Part model, mm, in its own coordinate system. Face numbers are marked on the shaded views. A direction names the side the tool comes from. Give positions to 0.01 mm unless a question says otherwise; leave off trailing zeros. Write each loop counter-clockwise with the first axis right and the second up, starting at its lowest first coordinate (ties: lowest second). Pieces come first, ordered by that corner, then holes.
from build123d import *

# Parameters (mm, degrees)
F2_DEPTH    = 10
F3_W        = 20.5154874287
F3_H        = 21.7
F4_DEPTH    = 1
F5_R        = 5
F7_T1_DEPTH = 14.7609215151
F7_T4_ANGLE = 34.9116466648
F7_T6_ANGLE = 279.6444662417
F7_T8_ANGLE = 34.9116520269


# Not quite as in the source:
# - a fillet or chamfer that OpenCascade refuses, or shapes differently, is made with other operations: its cross-section is extruded or revolved along the edge and cut away or added


with BuildPart() as f2:
    # F0 (on Top) → F2 (new body)
    with BuildSketch(Plane.XY):
        with BuildLine():
            ThreePointArc((7.5612498967, -5.5), (-9.35, 0), (7.5612498967, 5.5))
            Line((7.5612498967, 5.5), (8.2899034976, 7))
            ThreePointArc((8.2899034976, 7), (-10.85, 0), (8.2899034976, -7))
            Line((8.2899034976, -7), (7.5612498967, -5.5))
        make_face()
    extrude(amount=F2_DEPTH)

    # F3 (on Top) → F4 (join)
    with BuildSketch(Plane.XY):
        with Locations((-0.5922562857, 0)):
            Rectangle(F3_W, F3_H)
    extrude(amount=F4_DEPTH)

    # F5
    f5_edges = [f2.edges().sort_by_distance(p)[0] for p in [
        (-10.85, -10.85, 0.5),
        (9.665487, -10.85, 0.5),
        (-10.85, 10.85, 0.5),
        (9.665487, 10.85, 0.5),
    ]]
    fillet(f5_edges, radius=F5_R)

    # F7: fillet of radius 2 on 3 edges, made by hand

    # F7_s2 → F7_t1 (cut)
    with BuildSketch(Plane.XY.offset(1)):
        with BuildLine():
            ThreePointArc((8.2899034976, 7), (7.1091806232, 6.7248281543), (5.9864319049, 7.1822790985))
            ThreePointArc((5.9864319049, 7.1822790985), (6.8258652411, 6.3898406639), (7.5612498967, 5.5))
            Line((7.5612498967, 5.5), (8.2899034976, 7))
        make_face()
        with BuildLine():
            ThreePointArc((5.9864319049, -7.1822790985), (7.1091806232, -6.7248281543), (8.2899034976, -7))
            Line((8.2899034976, -7), (7.5612498967, -5.5))
            ThreePointArc((7.5612498967, -5.5), (6.8258652411, -6.3898406639), (5.9864319049, -7.1822790985))
        make_face()
    extrude(amount=F7_T1_DEPTH, mode=Mode.SUBTRACT)

    # F7_s3 → F7_t4 (revolve, cut)
    with BuildSketch(Plane(origin=(0, 0, 0), x_dir=(0, 0, 1), z_dir=(0.091781739, 0.9957791484, 0))):
        with BuildLine():
            ThreePointArc((8, 9.35), (9.4142135624, 9.9357864376), (10, 11.35))
            Line((10, 11.35), (10, 9.35))
            Line((10, 9.35), (8, 9.35))
        make_face()
    revolve(axis=Axis((0, 0, 10), (0, 0, -1)), revolution_arc=F7_T4_ANGLE, mode=Mode.SUBTRACT)

    # F7_s5 → F7_t6 (revolve, cut)
    with BuildSketch(Plane(origin=(0, 0, 0), x_dir=(0, 0, 1), z_dir=(0.6451612191, 0.7640464655, 0))):
        with BuildLine():
            ThreePointArc((8.0635083269, 9.35), (9.2882531983, 9.7688611699), (10, 10.85))
            Line((10, 10.85), (10, 9.35))
            Line((10, 9.35), (8.0635083269, 9.35))
        make_face()
    revolve(axis=Axis((0, 0, 10), (0, 0, -1)), revolution_arc=F7_T6_ANGLE, mode=Mode.SUBTRACT)

    # F7_s7 → F7_t8 (revolve, cut)
    with BuildSketch(Plane(origin=(0, 0, 0), x_dir=(0, 0, 1), z_dir=(-0.6451612906, 0.7640464051, 0))):
        with BuildLine():
            ThreePointArc((8, 9.35), (9.4142135624, 9.9357864376), (10, 11.35))
            Line((10, 11.35), (10, 9.35))
            Line((10, 9.35), (8, 9.35))
        make_face()
    revolve(axis=Axis((0, 0, 10), (0, 0, -1)), revolution_arc=F7_T8_ANGLE, mode=Mode.SUBTRACT)


solid = f2.part
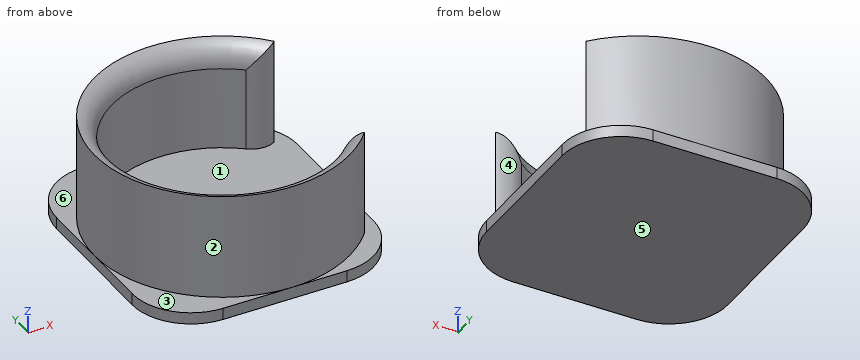
1) Saw through at B-B (z = 9.25). Write the cut outline in (x, y), and give its area (3 significant figures).
Check result:
outline: (7.04, -6.73) arc R9.74 cw (long way) to (7.04, 6.73) arc R2 ccw to (8.29, 7) arc R10.85 ccw (long way) to (8.29, -7) arc R2 ccw to start
area: 55.3 mm2
2) Flat gauge pins, fed straight in: P1, Ø3.5, axis at x = -7, y = 4, coming from the +Z side; P2, Ø1, axis at x = 2.5, z = 7, coming from the -Y side; P3, Ø1.5, axis at y = -4.5, z = 6.5, coming from the -X side. Where does each tip first touch, or does it go through?
Check result:
P1: stops at z = 9.34
P2: stops at y = -10.66
P3: stops at x = -10.18
3) Mould opens along Y. For the marked faces 1, 2 and 3 say: +Y half, -Y half, draft (parallel to the pull), parting line (faces both ways), or undercut.
Check result:
face 1: undercut
face 2: parting line
face 3: draft
4) Drill centre lines: L1, parallel to Y at x = 0, z = 3.5; L2, parallel to X at y = 0, z = 4.75; L3, parallel to Z at x = 4.25, y = 0. Where is each one in solid material? Low to high.
Check result:
L1: y = -10.85 to -9.35, 9.35 to 10.85
L2: x = -10.85 to -9.35
L3: z = 0 to 1
5) 3-axis set-ups, long thin cutter, end or side, ignore diameter. For the marked faces 4, 5 and 6: which of +Z, -Z, +X, -X, +Y, -Y reach the whole face in a straight line?
Check result:
face 4: +Z
face 5: -Z, +X, -X, +Y, -Y
face 6: +Z, -X, +Y
6) Saw through at A-A (z = 5.25). Write the cut outline in (x, y), and give its area (3 significant figures).
Check result:
outline: (5.99, -7.18) arc R9.35 cw (long way) to (5.99, 7.18) arc R2 ccw to (8.29, 7) arc R10.85 ccw (long way) to (8.29, -7) arc R2 ccw to start
area: 72.7 mm2
